Design review of the part built by this model. Coordinates are the model's own, in mm. A direction names the side the tool comes from. Give positions to 0.01 mm unless a question says otherwise; leave off trailing zeros. Write each loop counter-clockwise with the first axis right and the second up, starting at its lowest first coordinate (ties: lowest second). Pieces come first, ordered by that corner, then holes. Notation, with made-up numbers: (66.25, -24) -> (108.25, -24) arc R33 ccw to (108.25, 10) -> close; hole circle Ø11 at (62, 82.25). An arc over 180 degrees is marked (long way). Return JSON: item names as keys, results as strings. Group by question number.
from build123d import *

# Parameters (mm, degrees)
F1_DEPTH = 40
F2_R     = 1.55
F3_DEPTH = 4


with BuildPart() as f1:
    # F0 (on Front) → F1 (new body)
    with BuildSketch(Plane.XZ):
        Polygon((50, 0), (0, 0), (0, -35), (4, -35), (4, -4), (50, -4), align=None)
    extrude(amount=F1_DEPTH)

    # F2 (on face) → F3 (cut, through all)
    with BuildSketch(Plane.XY):
        with Locations((45, -10)):
            Circle(F2_R)
        with Locations((45, -30)):
            Circle(F2_R)
    extrude(amount=-F3_DEPTH, mode=Mode.SUBTRACT)


solid = f1.part
Q1. Take a section at D-D, the plane y = -35. Give the boundary of the cut face in (x, z), plus the area to 3 significant figures.
Q2. Tool access review of faces 1 (the face through (14, -40, -3)), 2 (the face through (27, -20, -4)): name each direction out of +Z, -Z, +X, -X, +Y, -Y from which nothing blocks a thin tool from reaching the whole face with its end or side.
Q3. For L1, parallel to Y at x = 45, z = -3; L2, parallel to Z at x = 40.5, y = -36.5; L3, parallel to X at y = -12.5, z = -20, list the stretches that pass through material, from the lowest coordinate up. Write a range as from..to.
Q4. Mouldability with a two-part tool opening along Y and no side actions: class faces 3 (the face through (14, 0, -3)), 4 (the face through (46.478, -29.534, -1.972)), 5 (the face through (0, -20, -17)) as +Y half, -Y half, draft (parallel to the pull), parting line (faces both ways), or undercut.
Q5. Take a section at A-A, the plane x = 45. Give the boundary of the cut face in (y, z), plus the area to 3 significant figures.
Q6. Take a section at C-C, the plane x = 18. Give the boundary of the cut face in (y, z), plus the area to 3 significant figures.
Q7. Take a section at B-B, the plane y = -30. Give the boundary of the cut face in (x, z).
Q8. Insertion check: pin 1 (6 mm diameter, centred on y = -17.5, z = -29.5, fed in from -X); pin 2 (4 mm diameter, centred on x = 14, y = -15.5, fed in from -Z). Each pin has a flat end and moves straight along its axis. Give the tip position at first contact, or say it passes through.
Final values:
{
 "1": {"outline": "(0, -35) -> (4, -35) -> (4, -4) -> (50, -4) -> (50, 0) -> (0, 0) -> close", "area": "324 mm²"},
 "2": {"face 1": "+Z, -Z, +X, -X, -Y", "face 2": "-Z, +X, +Y, -Y"},
 "3": {"L1": "y = -40..-31.55, -28.45..-11.55, -8.45..0", "L2": "z = -4..0", "L3": "x = 0..4"},
 "4": {"face 3": "+Y half", "face 4": "undercut", "face 5": "draft"},
 "5": {"outline": "(-40, -4) -> (-31.55, -4) -> (-31.55, 0) -> (-40, 0) -> close; (-28.45, -4) -> (-11.55, -4) -> (-11.55, 0) -> (-28.45, 0) -> close; (-8.45, -4) -> (0, -4) -> (0, 0) -> (-8.45, 0) -> close", "area": "135 mm²"},
 "6": {"outline": "(-40, -4) -> (0, -4) -> (0, 0) -> (-40, 0) -> close", "area": "160 mm²"},
 "7": {"outline": "(0, -35) -> (4, -35) -> (4, -4) -> (43.45, -4) -> (43.45, 0) -> (0, 0) -> close; (46.55, -4) -> (50, -4) -> (50, 0) -> (46.55, 0) -> close"},
 "8": {"pin 1": "stops at x = 0", "pin 2": "stops at z = -4"}
}
